Design review of the part built by this model. Coordinates are the model's own, in mm. A direction names the side the tool comes from. Give positions to 0.01 mm unless a question says otherwise; leave off trailing zeros. Write each loop counter-clockwise with the first axis right and the second up, starting at its lowest first coordinate (ties: lowest second). Pieces come first, ordered by that corner, then holes. Notation, with made-up numbers: M 8,77.5 L 59,77.5 A23 cw 59,102.5 Z; hole C 43.5,74.25 d10. An arc over 180 degrees is marked long. Answer in a Markdown table with one row per item.
```python
from build123d import *

# Parameters (mm, degrees)
ESQUISSE1_W             = 88.22
ESQUISSE1_H             = 50
BOSS_EXTRU_2_DEPTH      = 18.22
ESQUISSE3_W             = 38
ESQUISSE3_H             = 50
ENL_V_MAT_EXTRU_1_DEPTH = 10
ESQUISSE6_W             = 58
ESQUISSE6_H             = 18.22
ENL_V_MAT_EXTRU_2_DEPTH = 5
ESQUISSE7_W             = 58
ESQUISSE7_H             = 18.22
ENL_V_MAT_EXTRU_3_DEPTH = 5
CONG_6_R                = 5
CONG_11_R               = 5
ESQUISSE8_R             = 17.5
ENL_V_MAT_EXTRU_4_DEPTH = 92.952500984
ESQUISSE10_W            = 38
ESQUISSE10_H            = 20
ENL_V_MAT_EXTRU_5_DEPTH = 92.952500984
CONG_7_R                = 5
CONG_8_R                = 5
CONG_9_R                = 5
CONG_10_R               = 5
ESQUISSE11_R            = 4
ENL_V_MAT_EXTRU_6_DEPTH = 92.952500984


with BuildPart() as part:
    # Esquisse1 → Boss.-Extru.2 (new body)
    with BuildSketch(Plane(origin=(0, 0, 0), x_dir=(1, 0, 0), z_dir=(0, 1, 0))):
        with Locations((20.751905501, -37.579767114)):
            Rectangle(ESQUISSE1_W, ESQUISSE1_H)
    extrude(amount=BOSS_EXTRU_2_DEPTH)

    # Esquisse3 → Enlèv. mat.-Extru.1 (cut)
    with BuildSketch(Plane(origin=(0, 0, 0), x_dir=(-1, 0, 0), z_dir=(0, -1, 0))):
        with Locations((-25.861905501, -37.579767114)):
            Rectangle(ESQUISSE3_W, ESQUISSE3_H)
    extrude(amount=-ENL_V_MAT_EXTRU_1_DEPTH, mode=Mode.SUBTRACT)

    # Esquisse6 → Enlèv. mat.-Extru.2 (cut)
    with BuildSketch(Plane.XY.offset(62.579767114)):
        with Locations((35.861905501, 9.11)):
            Rectangle(ESQUISSE6_W, ESQUISSE6_H)
    extrude(amount=-ENL_V_MAT_EXTRU_2_DEPTH, mode=Mode.SUBTRACT)

    # Esquisse7 → Enlèv. mat.-Extru.3 (cut)
    with BuildSketch(Plane(origin=(0, 0, 12.579767114), x_dir=(-1, 0, 0), z_dir=(0, 0, -1))):
        with Locations((-35.861905501, 9.11)):
            Rectangle(ESQUISSE7_W, ESQUISSE7_H)
    extrude(amount=-ENL_V_MAT_EXTRU_3_DEPTH, mode=Mode.SUBTRACT)

    # Congé6
    cong_6_edges = [part.edges().sort_by_distance(p)[0] for p in [
        (6.861905501, 14.11, 17.579767114),
    ]]
    fillet(cong_6_edges, radius=CONG_6_R - 0.0001)  # a hair under: the kernel refuses the full size

    # Congé11
    cong_11_edges = [part.edges().sort_by_distance(p)[0] for p in [
        (6.861905501, 14.11, 57.579767114),
    ]]
    fillet(cong_11_edges, radius=CONG_11_R - 0.0001)  # a hair under: the kernel refuses the full size

    # Esquisse8 → Enlèv. mat.-Extru.4 (cut, through all)
    with BuildSketch(Plane(origin=(0, 18.22, 0), x_dir=(1, 0, 0), z_dir=(0, 1, 0))):
        with Locations((-23.358094499, -37.579767114)):
            Circle(ESQUISSE8_R)
    extrude(amount=-ENL_V_MAT_EXTRU_4_DEPTH, mode=Mode.SUBTRACT)

    # Esquisse10 → Enlèv. mat.-Extru.5 (cut, through all)
    with BuildSketch(Plane(origin=(0, 18.22, 0), x_dir=(1, 0, 0), z_dir=(0, 1, 0))):
        with Locations((25.861905501, -37.579767114)):
            Rectangle(ESQUISSE10_W, ESQUISSE10_H)
    extrude(amount=-ENL_V_MAT_EXTRU_5_DEPTH, mode=Mode.SUBTRACT)

    # Congé7
    cong_7_edges = [part.edges().sort_by_distance(p)[0] for p in [
        (6.861905501, 14.11, 27.579767114),
    ]]
    fillet(cong_7_edges, radius=CONG_7_R)

    # Congé8
    cong_8_edges = [part.edges().sort_by_distance(p)[0] for p in [
        (6.861905501, 14.11, 47.579767114),
    ]]
    fillet(cong_8_edges, radius=CONG_8_R)

    # Congé9
    cong_9_edges = [part.edges().sort_by_distance(p)[0] for p in [
        (44.861905501, 14.11, 27.579767114),
    ]]
    fillet(cong_9_edges, radius=CONG_9_R)

    # Congé10
    cong_10_edges = [part.edges().sort_by_distance(p)[0] for p in [
        (44.861905501, 14.11, 47.579767114),
    ]]
    fillet(cong_10_edges, radius=CONG_10_R)

    # Esquisse11 → Enlèv. mat.-Extru.6 (cut, through all)
    with BuildSketch(Plane(origin=(0, 18.22, 0), x_dir=(1, 0, 0), z_dir=(0, 1, 0))):
        with Locations(Location((54.861905501, -49.579767114, 0), (0, 0, 270))):
            Circle(ESQUISSE11_R)
        with Locations(Location((54.861905501, -25.579767114, 0), (0, 0, 270))):
            Circle(ESQUISSE11_R)
    extrude(amount=-ENL_V_MAT_EXTRU_6_DEPTH, mode=Mode.SUBTRACT)


solid = part.part
```
1) Add section B-B (x = 34). Write out the cut boundary in (y, z).
Geometry says:
| item | result |
|---|---|
| outline | M 10,17.58 L 18.22,17.58 L 18.22,27.58 L 10,27.58 Z; M 10,47.58 L 18.22,47.58 L 18.22,57.58 L 10,57.58 Z |
2) Add section A-A (y = 5.25). Write out the cut boundary in (x, z), and give its area (3 significant figures).
Geometry says:
| item | result |
|---|---|
| outline | M -23.36,12.58 L 6.86,12.58 L 6.86,62.58 L -23.36,62.58 L -23.36,55.08 A17.5 cw -23.36,20.08 Z; M 44.86,17.58 L 64.86,17.58 L 64.86,57.58 L 44.86,57.58 Z; hole C 54.86,25.58 d8; hole C 54.86,49.58 d8 |
| area | 1,730 mm^2 |
3) Insertion check: P1, Ø5.5, axis at x = 41.5, y = 10, coming from the +Z side; P2, Ø12, axis at x = -5, z = 57.5, coming from the -Y side; P3, Ø2, axis at y = 15.5, z = 23, coming from the -X side; P4, Ø6, axis at x = 28, z = 53.5, coming from the -Y side. Each pin has a flat end and moves straight along its axis. Give the tip position at first contact, or say it passes through.
Geometry says:
| item | result |
|---|---|
| P1 | z = 57.58 |
| P2 | y = 0 |
| P3 | x = -15.39 |
| P4 | y = 10 |
4) The part is to be moulded in two halves that separate along X. For faces 5 (the face through (26, 14, 47.58)), 6 (the face through (44, 11, 57.58)), 7 (the face through (64.862, 9, 38)), say which applies: released by +X, released by -X, zero draft, split by the parting line, or undercut.
Geometry says:
| item | result |
|---|---|
| face 5 | undercut |
| face 6 | zero draft |
| face 7 | released by +X |
5) Add section D-D (x = 53.5). Write out the cut boundary in (y, z), and give its area (3 significant figures).
Geometry says:
| item | result |
|---|---|
| outline | M 0,17.58 L 18.22,17.58 L 18.22,21.82 L 0,21.82 Z; M 0,29.34 L 18.22,29.34 L 18.22,45.82 L 0,45.82 Z; M 0,53.34 L 18.22,53.34 L 18.22,57.58 L 0,57.58 Z |
| area | 455 mm^2 |
6) Add section C-C (z = 49). Write out the cut boundary in (x, y), and give its area (3 significant figures).
Geometry says:
| item | result |
|---|---|
| outline | M -10.1,0 L 6.86,0 L 6.86,10 L 44.86,10 L 44.86,0 L 50.9,0 L 50.9,18.22 L -10.1,18.22 Z; M 58.82,0 L 64.86,0 L 64.86,18.22 L 58.82,18.22 Z |
| area | 842 mm^2 |
7) For faces 1 (the face through (8.365, 14.052, 46.154)), 2 (the face through (44.862, 7, 38)), 3 (the face through (45, 11, 17.58)), 4 (the face through (26, 10, 52)), list the 3-axis set-ups (+Z, -Z, +X, -X, +Y, -Y) from which the entire face can be reached by the end or side of a thin tool; tool diameter is ignored.
Geometry says:
| item | result |
|---|---|
| face 1 | +Y, -Y |
| face 2 | -Y |
| face 3 | -Z, +X, +Y, -Y |
| face 4 | +Z, -Z, -Y |
8) To check wall thickness, follow probe 1 along X at (y, z) = (2, 23); probe 2 along Z at (x, y) = (-8, 16.25); probe 3 along X at (y, z) = (2.5, 25.5). State the ranges of each line that lie inside material, in increasing order. Write a range as [from, to].
Geometry says:
| item | result |
|---|---|
| probe 1 | [-13.68, 6.86], [44.86, 51.8], [57.92, 64.86] |
| probe 2 | [12.58, 29.19], [45.97, 62.58] |
| probe 3 | [-10.7, 6.86], [44.86, 50.86], [58.86, 64.86] |
